Autodesk Inventor part; units mm, degrees
ref_plane "YZ Plane" through (0, 0, 0) normal (1, 0, 0) x (0, 1, 0)
ref_plane "XZ Plane" through (0, 0, 0) normal (0, 1, 0) x (-1, 0, 0)
ref_plane "XY Plane" through (0, 0, 0) normal (0, 0, 1) x (1, 0, 0)
sketch "Sketch1" plane through (0, 0, 0) normal (0, 0, 1) x (1, 0, 0)
  circle A0 centre (16.5752, 43.5198) radius 1.65
  line L0 (21.3312, 42.5198) -> (19.4442, 39.2514)
  arc A1 (21.3312, 42.5198) -> (21.3312, 44.5198) centre (19.5992, 43.5198) ccw
  line L1 (19.8192, 47.1386) -> (21.3312, 44.5198)
  arc A2 (19.8192, 47.1386) -> (18.0872, 48.1386) centre (18.0872, 46.1386) ccw
  line L2 (15.0633, 48.1386) -> (18.0872, 48.1386)
  arc A3 (15.0633, 48.1386) -> (13.3312, 47.1386) centre (15.0633, 46.1386) ccw
  line L3 (11.8192, 44.5198) -> (13.3312, 47.1386)
  arc A4 (11.8192, 44.5198) -> (11.8192, 42.5198) centre (13.5513, 43.5198) ccw
  line L4 (13.7915, 39.1038) -> (11.8192, 42.5198)
  line L5 (13.7915, 39.1038) -> (13.7915, 1.2514)
  line L6 (13.7915, 1.2514) -> (79.2915, 1.2514)
  line L7 (79.2915, 1.2514) -> (79.2915, 39.2514)
  line L8 (79.2915, 39.2514) -> (19.4442, 39.2514)
  point P0 (0, 0)
  point P1 (0, 0)
  dimension "d0" = 65.5
  dimension "d1" = 38
  dimension "d3" = 37.8524
  dimension "d4" = 90
  dimension "d5" = 90
  dimension "d6" = 5.6528
  dimension "d10" = 90
extrude "Extrusion1" add sketch "Sketch1" along normal blind 1.5
sketch "Sketch2" plane through (0, 0, 0) normal (0, 0, -1) x (-1, 0, 0)
  circle A0 centre (-16.5752, 43.5198) radius 1.65
  line L0 (-13.7915, 1.2514) -> (-13.7915, 39.1038)
  line L1 (-13.7915, 39.1038) -> (-11.8192, 42.5198)
  arc A1 (-11.8192, 42.5198) -> (-11.8192, 44.5198) centre (-13.5513, 43.5198) ccw
  line L2 (-11.8192, 44.5198) -> (-13.3312, 47.1386)
  arc A2 (-13.3312, 47.1386) -> (-15.0633, 48.1386) centre (-15.0633, 46.1386) ccw
  line L3 (-15.0633, 48.1386) -> (-18.0872, 48.1386)
  arc A3 (-18.0872, 48.1386) -> (-19.8192, 47.1386) centre (-18.0872, 46.1386) ccw
  line L4 (-19.8192, 47.1386) -> (-21.3312, 44.5198)
  arc A4 (-21.3312, 44.5198) -> (-21.3312, 42.5198) centre (-19.5992, 43.5198) ccw
  line L5 (-21.3312, 42.5198) -> (-19.4442, 39.2514)
  line L6 (-19.4442, 39.2514) -> (-79.2915, 39.2514)
  line L7 (-79.2915, 39.2514) -> (-79.2915, 1.2514)
  line L8 (-79.2915, 1.2514) -> (-13.7915, 1.2514)
  line L9 (-77.7629, 37.2514) -> (-15.7915, 37.2514)
  line L10 (-15.7915, 37.2514) -> (-15.7915, 3.2514)
  line L11 (-15.7915, 3.2514) -> (-77.7629, 3.2514)
  line L12 (-77.7629, 37.2514) -> (-79.2915, 37.2514)
  line L13 (-77.7629, 3.2514) -> (-79.2915, 3.2514)
  point P0 (0, 0)
  dimension "d11" = 2
  dimension "d12" = 2
  dimension "d13" = 2
extrude "Extrusion2" add sketch "Sketch2" against normal blind 6.5 contours L8 L7 L13 L11 L10 L9 L12 L6 L5 A4 L4 A3 L3 A2 L2 A1 L1 L0
sketch "Sketch3" plane through (0, 0, 0) normal (0, 0, -1) x (-1, 0, 0)
  line L0 (-79.2915, 39.2514) -> (-79.2915, 1.2514)
  line L1 (-19.4442, 39.2514) -> (-79.2915, 39.2514)
  line L2 (-71.2915, 33.2514) -> (-64.2915, 33.2514)
  line L3 (-64.2915, 33.2514) -> (-64.2915, 29.7514)
  line L4 (-64.2915, 29.7514) -> (-71.2915, 29.7514)
  line L5 (-71.2915, 29.7514) -> (-71.2915, 33.2514)
  circle A0 centre (-71.2915, 31.5014) radius 1.75
  circle A1 centre (-64.2915, 31.5014) radius 1.75
  point P0 (0, 0)
  dimension "d16" = 3.5
  dimension "d17" = 7
  dimension "d18" = 6
  dimension "d19" = 8
extrude "Extrusion3" cut sketch "Sketch3" against normal blind 2.5
pattern_linear "Rectangular Pattern1" count 4 spacing 15 along (-1, 0, 0) count 3 spacing 10 along (0, -1, 0) of "Extrusion3"
properties part number "case add on sdr top"
Source: CAD feature listing. Evaluate the final solid. Frame: model axes, mm. A direction names the side the tool comes from. Give positions to 0.01 mm unless a question says otherwise; leave off trailing zeros. Loops run counter-clockwise (first coordinate to the right, second up) from the corner with the lowest first, then second, coordinate; pieces in that order, holes last. Notation, with made-up numbers: (-27.5, 87.5) -> (-20.5, 87.5) arc R22 ccw to (-20.5, 111.5) -> close; hole circle Ø11 at (69.25, 61.25). An arc over 180 degrees is marked (long way). Use a Markdown table: item, result. Add a question column.
(1) Access query for faces 1 (the face through (68, 9.751, 1)), 2 (the face through (12.565, 45.811, 3.204)), 3 (the face through (47, 3.251, 4)). Directions: +Z, -Z, +X, -X, +Y, -Y. A direction counts if a zero-diameter tool reaches every point of the face in a straight line with its end or side. Return the directions, or none.
(2) Section query C-C (z = 4.25). Output: boundary loops of the cut face in (x, y).
(3) Section query B-B (y = 12.5). Output: boundary loops of the cut face in (x, z), then the cut area to 3 significant figures.
(4) Pull-direction query (Y, two-part tool) for faces 4 (the face through (20.565, 45.848, 3.204)), 5 (the face through (68, 23.251, 1)); classes: +Y half, -Y half, draft (parallel to the pull), parting line (faces both ways), or undercut.
(5) Ray query, line 1 (Y direction, x = 53, z = 0.75); line 2 (Y direction, x = 52.5, z = 4.5); line 3 (Y direction, x = 56.5, z = 1.25). Return the intervals inside material, ascending.
(6) Section query A-A (x = 35). Output: boundary loops of the cut face in (y, z).
(7) Section query D-D (x = 59.5). Output: boundary loops of the cut face in (y, z), then the cut area to 3 significant figures.
(8) First-contact query: pin 1 Ø5.5 at (x, y) = (16.58, 43.52) entering from -Z; pin 2 Ø1.6 at (x, z) = (68, 1) entering from +Y; pin 3 Ø3 at (y, z) = (26, 4) entering from -X. Flat tips, straight axial feed; report the tip coordinate or a pass-through.
Checked values:
| question | item | result |
|---|---|---|
| 1 | face 1 | +Z, -Z |
| 1 | face 2 | +Z, -Z, -X, +Y |
| 1 | face 3 | +Z, +X |
| 2 | outline | (11.82, 42.52) -> (13.79, 39.1) -> (13.79, 1.25) -> (79.29, 1.25) -> (79.29, 3.25) -> (15.79, 3.25) -> (15.79, 37.25) -> (79.29, 37.25) -> (79.29, 39.25) -> (19.44, 39.25) -> (21.33, 42.52) arc R2 ccw to (21.33, 44.52) -> (19.82, 47.14) arc R2 ccw to (18.09, 48.14) -> (15.06, 48.14) arc R2 ccw to (13.33, 47.14) -> (11.82, 44.52) arc R2 ccw to start; hole circle Ø3.3 at (16.58, 43.52) |
| 3 | outline | (13.79, 0) -> (17.85, 0) -> (17.85, 1.5) -> (15.79, 1.5) -> (15.79, 6.5) -> (13.79, 6.5) -> close; (27.73, 0) -> (32.85, 0) -> (32.85, 1.5) -> (27.73, 1.5) -> close; (42.73, 0) -> (47.85, 0) -> (47.85, 1.5) -> (42.73, 1.5) -> close; (57.73, 0) -> (62.85, 0) -> (62.85, 1.5) -> (57.73, 1.5) -> close; (72.73, 0) -> (79.29, 0) -> (79.29, 1.5) -> (72.73, 1.5) -> close |
| 3 | area | 49.0 mm^2 |
| 4 | face 4 | +Y half |
| 4 | face 5 | undercut |
| 5 | line 1 | 1.25 to 9.75, 13.25 to 19.75, 23.25 to 29.75, 33.25 to 39.25 |
| 5 | line 2 | 1.25 to 3.25, 37.25 to 39.25 |
| 5 | line 3 | 1.25 to 9.76, 13.24 to 19.76, 23.24 to 29.76, 33.24 to 39.25 |
| 6 | outline | (1.25, 0) -> (9.75, 0) -> (9.75, 1.5) -> (3.25, 1.5) -> (3.25, 6.5) -> (1.25, 6.5) -> close; (13.25, 0) -> (19.75, 0) -> (19.75, 1.5) -> (13.25, 1.5) -> close; (23.25, 0) -> (29.75, 0) -> (29.75, 1.5) -> (23.25, 1.5) -> close; (33.25, 0) -> (39.25, 0) -> (39.25, 6.5) -> (37.25, 6.5) -> (37.25, 1.5) -> (33.25, 1.5) -> close |
| 7 | outline | (1.25, 0) -> (39.25, 0) -> (39.25, 6.5) -> (37.25, 6.5) -> (37.25, 1.5) -> (3.25, 1.5) -> (3.25, 6.5) -> (1.25, 6.5) -> close |
| 7 | area | 77.0 mm^2 |
| 8 | pin 1 | z = 0 |
| 8 | pin 2 | y = 39.25 |
| 8 | pin 3 | x = 13.79 |
